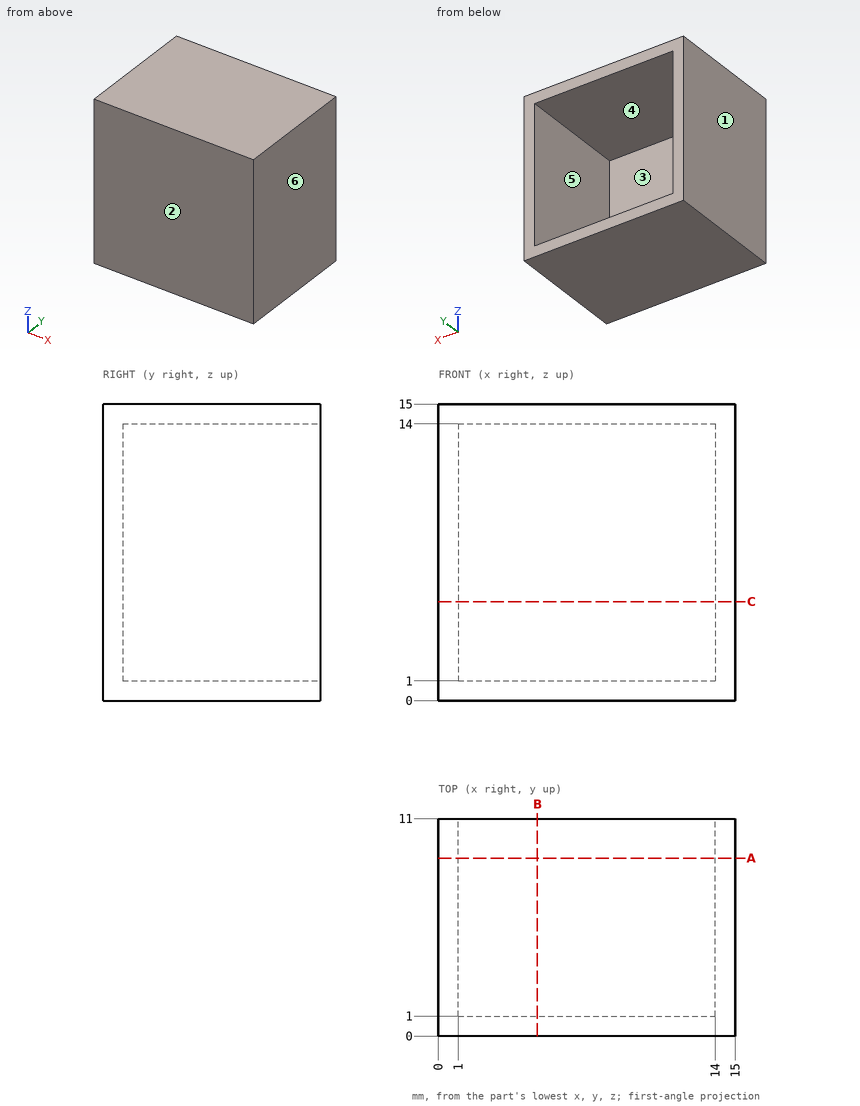
Can you work these out from the drawing? Everything is in mm from the part's minimum corner. A direction names the side the tool comes from. Round coordinates to 2 decimals unless told otherwise and drop trailing zeros. Loops run counter-clockwise (first coordinate to the right, second up) from the corner with the lowest first, then second, coordinate; pieces in that order, holes last. Notation, with made-up numbers: (-22.5, 68) - (24.5, 68) arc R26 cw to (24.5, 95) - close; hole circle Ø7 at (64, 60.25). An arc over 180 degrees is marked (long way). One line per question, with ' | ' between items. Start each with the question number.
Q1. I want a section at B-B (x = 5). Write out the boundary of the cut face in (y, z), then the cut area to 3 significant figures.
Q2. Will these pins go through, and if not, where does the flat tip stop? pin 1 (3 mm diameter, centred on x = 8.5, y = 4.5, fed in from -Z); pin 2 (1.5 mm diameter, centred on x = 12.5, z = 11.5, fed in from +Y).
Q3. I want a section at C-C (z = 5). Write out the boundary of the cut face in (x, y).
Q4. I want a section at A-A (y = 9). Write out the boundary of the cut face in (x, z).
Q5. For the marked faces 5 and 6, which set-ups out of +Z, -Z, +X, -X, +Y, -Y let a thin tool reach every point of the face, with its end or its side?
Q6. Please list where these lines run through material, in increasing order: line 1 (Z direction, x = 6.5, y = 6); line 2 (Y direction, x = 10, z = 11.5). Write a range as [from, to].
Q7. We'd pull the mould along X, two halves only. Please class the marked faces 1, 2, 3 and 4: +X half, -X half, draft (parallel to the pull), parting line (faces both ways), or undercut.
Response values:
1) outline: (0, 0) - (11, 0) - (11, 1) - (1, 1) - (1, 14) - (11, 14) - (11, 15) - (0, 15) - close | area: 35.0 mm²
2) pin 1: stops at z = 0 | pin 2: stops at y = 1
3) outline: (0, 0) - (15, 0) - (15, 11) - (14, 11) - (14, 1) - (1, 1) - (1, 11) - (0, 11) - close
4) outline: (0, 0) - (15, 0) - (15, 15) - (0, 15) - close; hole (1, 1) - (14, 1) - (14, 14) - (1, 14) - close
5) face 5: +Y | face 6: +Z, -Z, +X, +Y, -Y
6) line 1: z = [0, 1], [14, 15] | line 2: y = [0, 1]
7) face 1: -X half | face 2: draft | face 3: undercut | face 4: undercut
